The listing builds one solid part. Answer for the finished solid, in the listing's coordinates (mm). A direction names the side the tool comes from. Coordinates: 2 decimals unless noted, no trailing zeros. Loops run counter-clockwise (first coordinate to the right, second up) from the corner with the lowest first, then second, coordinate; pieces in that order, holes last. Notation, with made-up numbers: (78.5, 26.25) - (103.5, 26.25) arc R22 cw to (103.5, 44.25) - close; hole circle Ø5 at (69, -19). An arc over 180 degrees is marked (long way). Put each result on its own line as item: value.
```python
from build123d import *

# Parameters (mm, degrees)
SKETCH_1_W          = 12
SKETCH_1_H          = 12
EXTRUDE_1_DEPTH     = 4
EXTRUDE_2_DEPTH     = 12
CUT_EXTRUDE_3_DEPTH = 29.587584718
SKETCH_5_W          = 7.4
SKETCH_5_H          = 12
EXTRUDE_3_DEPTH     = 0.4
SKETCH_3_R          = 2.6
CUT_EXTRUDE_1_DEPTH = 28.299267389
SKETCH_4_R          = 5
CUT_EXTRUDE_2_DEPTH = 28.299267389
FILLET_1_R          = 2.5


with BuildPart() as part:
    # Эскиз1 → Бобышка-Вытянуть1 (new body)
    with BuildSketch(Plane.XY):
        with Locations((6, 6)):
            Rectangle(SKETCH_1_W, SKETCH_1_H)
    extrude(amount=EXTRUDE_1_DEPTH)

    # Эскиз2 → Бобышка-Вытянуть2 (add)
    with BuildSketch(Plane(origin=(0, 12, 0), x_dir=(1, 0, 0), z_dir=(0, 1, 0))):
        with BuildLine():
            Line((8.5, 0), (23.5, 0))
            Line((23.5, 0), (23.5, -3.5))
            ThreePointArc((23.5, -3.5), (16, -11), (8.5, -3.5))
            Line((8.5, -3.5), (8.5, 0))
        make_face()
    extrude(amount=-EXTRUDE_2_DEPTH)

    # Эскиз6 → Вырез-Вытянуть3 (cut, through all)
    with BuildSketch(Plane(origin=(0, 12, 0), x_dir=(1, 0, 0), z_dir=(0, 1, 0))):
        with BuildLine():
            Line((11.5, -3.5), (11.5, 0))
            Line((11.5, 0), (20.5, 0))
            Line((20.5, 0), (20.5, -3.5))
            ThreePointArc((20.5, -3.5), (16, -8), (11.5, -3.5))
        make_face()
    extrude(amount=-CUT_EXTRUDE_3_DEPTH, mode=Mode.SUBTRACT)

    # Эскиз5 → Бобышка-Вытянуть3 (add)
    with BuildSketch(Plane(origin=(0, 0, 0), x_dir=(-1, 0, 0), z_dir=(0, 0, -1))):
        with Locations((-5.75, 6)):
            Rectangle(SKETCH_5_W, SKETCH_5_H)
    extrude(amount=EXTRUDE_3_DEPTH)

    # Эскиз3 → Вырез-Вытянуть1 (cut, through all)
    with BuildSketch(Plane.XY.offset(4)):
        with Locations((5.75, 6)):
            Circle(SKETCH_3_R)
    extrude(amount=-CUT_EXTRUDE_1_DEPTH, mode=Mode.SUBTRACT)

    # Эскиз4 → Вырез-Вытянуть2 (cut, through all)
    with BuildSketch(Plane.XY.offset(4)):
        with Locations((5.75, 6)):
            Circle(SKETCH_4_R)
    extrude(amount=CUT_EXTRUDE_2_DEPTH, mode=Mode.SUBTRACT)

    # Скругление1
    fillet_1_edges = [part.edges().sort_by_distance(p)[0] for p in [
        (0, 12, 2),
        (0, 0, 2),
    ]]
    fillet(fillet_1_edges, radius=FILLET_1_R)


solid = part.part
```
1) The part is cut by section C-C (x = 5.75). Give the vertices of the cut face in (y, z).
Found:
outline: (0, -0.4) - (3.4, -0.4) - (3.4, 4) - (0, 4) - close; (8.6, -0.4) - (12, -0.4) - (12, 4) - (8.6, 4) - close
2) Each of these flat-tipped pins is pushed along its axis until it touches: pin 1 (3 mm diameter, centred on y = 3.5, z = 5.5, fed in from +X); pin 2 (5 mm diameter, centred on x = 17.5, z = 3, fed in from +Y); pin 3 (2 mm diameter, centred on x = 20, y = 3.5, fed in from -Z); pin 4 (3 mm diameter, centred on y = 4.5, z = 8.5, fed in from +X). Where does it stop, or does it pass through?
Found:
pin 1: stops at x = 23.48
pin 2: passes through
pin 3: stops at z = 0
pin 4: stops at x = 22.63
3) For a pull along Y with two mould halves and no side action, classify faces 1 (the face through (2.9, 6.1, 4)), 2 (the face through (0.752, 0.713, 1.831)), 3 (the face through (6, 9, -0.4)) as pulls with the +Y half, pulls with the -Y half, needs draft (parallel to the pull), parting line crosses it, or undercut.
Found:
face 1: undercut
face 2: pulls with the -Y half
face 3: needs draft
4) Straight lines are drawn through the part: L1, parallel to X at y = 2.75, z = 0.5; L2, parallel to Z at x = 4.5, y = 3.25; L3, parallel to Y at x = 5.75, z = 2.85. For each, find the intervals that lie inside material, in ascending order. Write a range as [from, to].
Found:
L1: x = [0, 11.5], [20.5, 23.5]
L2: z = [-0.4, 4]
L3: y = [0, 3.4], [8.6, 12]
5) The part is cut by section A-A (z = 1.5). Give the vertices of the cut face in (x, y).
Found:
outline: (0, 2.5) arc R2.5 ccw to (2.5, 0) - (11.5, 0) - (11.5, 12) - (2.5, 12) arc R2.5 ccw to (0, 9.5) - close; (20.5, 0) - (23.5, 0) - (23.5, 12) - (20.5, 12) - close; hole circle Ø5.2 at (5.75, 6)
6) The part is cut by section B-B (y = 6). Give the vertices of the cut face in (x, z), and give its area (3 significant figures).
Found:
outline: (0, 0) - (2.05, 0) - (2.05, -0.4) - (3.15, -0.4) - (3.15, 4) - (0, 4) - close; (8.35, -0.4) - (9.45, -0.4) - (9.45, 0) - (11.5, 0) - (11.5, 3.5) arc R4.5 cw to (20.5, 3.5) - (20.5, 0) - (23.5, 0) - (23.5, 3.5) arc R7.5 ccw to (10.75, 8.86) - (10.75, 4) - (8.35, 4) - close
area: 84.4 mm^2
7) For faces 4 (the face through (11.5, 6, 2)), 5 (the face through (10.75, 5.93, 5.85)), 6 (the face through (1, 6, 0)), determine the directions among +Z, -Z, +X, -X, +Y, -Y from which every point of the face is accessible in a straight line to the end or side of a thin tool.
Found:
face 4: -Z, +Y, -Y
face 5: +Z, -X
face 6: -Z, -X, +Y, -Y
8) The part is cut by section D-D (z = 5.75). Give the vertices of the cut face in (x, y), and give its area (3 significant figures).
Found:
outline: (8.85, 0) - (12.1, 0) - (12.1, 12) - (8.85, 12) - (8.85, 9.93) arc R5 cw to (8.85, 2.07) - close; (19.9, 0) - (23.15, 0) - (23.15, 12) - (19.9, 12) - close
area: 67.8 mm^2
